```python
from build123d import *

# Parameters (mm, degrees)
SKETCH076_R      = 7.3
EXTRUDE077_DEPTH = 1.2
SKETCH074_R      = 1.8
SKETCH074_R_2    = 6.3
EXTRUDE076_DEPTH = 2


with BuildPart() as obj1:
    # Sketch076 → Extrude077 (new body)
    with BuildSketch(Plane.XZ):
        with Locations((-65, 21.2)):
            Circle(SKETCH076_R)
        with Locations((-42, 21.2)):
            Circle(SKETCH076_R)
        with Locations((-19, 21.2)):
            Circle(SKETCH076_R)
    extrude(amount=-EXTRUDE077_DEPTH)


with BuildPart() as cut044:
    # Sketch074 → Extrude076 (new body)
    with BuildSketch(Plane.XZ):
        with BuildLine():
            Line((-82.8, 3.2), (0, 3.2))
            Line((0, 3.2), (0, 39.2))
            Line((-195.886839, 39.2), (0, 39.2))
            Line((-202.764796, 20.302968), (-195.886839, 39.2))
            ThreePointArc((-192.175575, -3.18451), (-192.085048, 10.987093), (-202.764796, 20.302968))
            Line((-192.175575, -3.18451), (-215.419579, -53.031439))
            ThreePointArc((-215.419579, -53.031439), (-218.578907, -66.677212), (-215.93199, -80.431568))
            Line((-215.93199, -80.431568), (-176.68528, -80.431568))
            Line((-147.645309, 8.944272), (-176.68528, -80.431568))
            ThreePointArc((-132.428405, 20), (-141.832969, 16.944272), (-147.645309, 8.944272))
            Line((-132.428405, 20), (-107.6, 20))
            ThreePointArc((-91.751972, 6.2), (-97.09286, 16.066483), (-107.6, 20))
            Line((-82.8, 6.2), (-91.751972, 6.2))
            Line((-82.8, 3.2), (-82.8, 6.2))
        make_face()
        with Locations((-213.443268, -76.831568)):
            Circle(SKETCH074_R, mode=Mode.SUBTRACT)
        with Locations((-179.304663, -76.831568)):
            Circle(SKETCH074_R, mode=Mode.SUBTRACT)
        with Locations((-184.079668, 34.8)):
            Circle(SKETCH074_R, mode=Mode.SUBTRACT)
        with Locations((-78.51, 34.8)):
            Circle(SKETCH074_R, mode=Mode.SUBTRACT)
        with Locations((-78.51, 7.6)):
            Circle(SKETCH074_R, mode=Mode.SUBTRACT)
        with Locations((-5.6, 34.8)):
            Circle(SKETCH074_R, mode=Mode.SUBTRACT)
        with Locations((-5.6, 7.6)):
            Circle(SKETCH074_R, mode=Mode.SUBTRACT)
        with Locations((-19, 21.2)):
            Circle(SKETCH074_R_2, mode=Mode.SUBTRACT)
        with Locations((-42, 21.2)):
            Circle(SKETCH074_R_2, mode=Mode.SUBTRACT)
        with Locations((-65, 21.2)):
            Circle(SKETCH074_R_2, mode=Mode.SUBTRACT)
        Polygon((-189.938695, 31.567195), (-192.332836, 24.989347), (-196.467483, 26.494236), (-194.073342, 33.072084), (-193.885404, 33.00368), (-190.126633, 31.635599), align=None, mode=Mode.SUBTRACT)
    extrude(amount=-EXTRUDE076_DEPTH)

    # Cut044: cut obj1
    add(obj1.part, mode=Mode.SUBTRACT)


solid = cut044.part
```
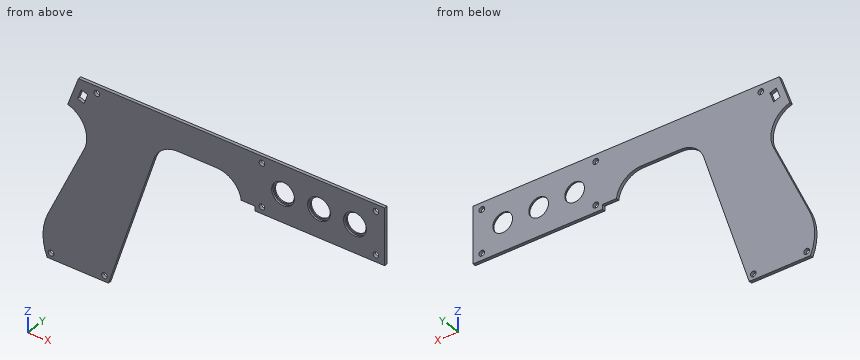
The model under review builds one solid part; all positions refer to its coordinate system, in mm. Give positions to 0.01 mm unless a question says otherwise; leave off trailing zeros. Write each loop counter-clockwise with the first axis right and the second up, starting at its lowest first coordinate (ties: lowest second). Pieces come first, ordered by that corner, then holes.
(1) To check wall thickness, follow L1, parallel to Z at x = -42, y = 0.35; L2, parallel to X at y = 1.85, z = 34.5; L3, parallel to Z at x = -35, y = 1.85. State the ranges of each line that lie inside material, in increasing order.
(2) For P1, Ø11.5, axis at x = -19, z = 21.2, coming from the -Y side; P2, Ø4.5, axis at x = -78.51, z = 7.6, coming from the +Y side; P3, Ø7.5, axis at x = -21, z = 18.5, coming from the -Y side, all flat-tipped, find the tip position at first contact; note any pin that passes through.
(3) Consider section A-A, the plane x = -42. Give the boundary of the cut face in (y, z).
(4) Consider section D-D, the plane z = -64. Give the boundary of the cut face in (x, y), and give its area (3 significant figures).
(5) Consider section C-C, the plane x = -113. Give the boundary of the cut face in (y, z).
(6) Consider section B-B, the plane y = 0.4. Give the number of separate pieces and of enclosed holes in the cut face, and give its area (3 significant figures).
Returned:
1. L1: z = 3.2 to 13.9, 28.5 to 39.2
1. L2: x = -197.6 to -185.85, -182.3 to -80.28, -76.74 to -7.37, -3.83 to 0
1. L3: z = 3.2 to 39.2
2. P1: passes through
2. P2: stops at y = 2
2. P3: stops at y = 1.2
3. outline: (0, 3.2) - (2, 3.2) - (2, 14.9) - (1.2, 14.9) - (1.2, 13.9) - (0, 13.9) - close; (0, 28.5) - (1.2, 28.5) - (1.2, 27.5) - (2, 27.5) - (2, 39.2) - (0, 39.2) - close
4. outline: (-218.42, 0) - (-171.35, 0) - (-171.35, 2) - (-218.42, 2) - close
4. area: 94.2 mm2
5. outline: (0, 20) - (2, 20) - (2, 39.2) - (0, 39.2) - close
6. separate pieces: 1
6. enclosed holes: 11
6. area: 9,300 mm2
